Read the model definition and answer for the solid it produces. Units are mm, in the model's axes. A direction names the side the tool comes from. Round coordinates to 2 decimals unless told otherwise and drop trailing zeros. Loops run counter-clockwise (first coordinate to the right, second up) from the corner with the lowest first, then second, coordinate; pieces in that order, holes last. Notation, with made-up numbers: M -40,54.5 L 19,54.5 A20 cw 19,74.5 Z; hole C -31.5,71 d3. An arc over 180 degrees is marked long. Write each question's results on one line, items separated by ' | '.
from build123d import *

# Parameters (mm, degrees)
SALIENTE_EXTRUIR1_DEPTH = 97.7
CROQUIS2_W              = 6.35
CROQUIS2_H              = 85
SALIENTE_EXTRUIR2_DEPTH = 70
CORTAR_EXTRUIR1_DEPTH   = 120
CROQUIS4_R              = 37.5
CROQUIS4_R_2            = 3
CORTAR_EXTRUIR2_DEPTH   = 120
CROQUIS5_W              = 30
CROQUIS5_H              = 18.85
CORTAR_EXTRUIR3_DEPTH   = 120
REDONDEO1_R             = 1
CORTAR_EXTRUIR4_DEPTH   = 110


with BuildPart() as part:
    # Croquis1 → Saliente-Extruir1 (new body)
    with BuildSketch(Plane.XY):
        Polygon((34.307403189, -10.15), (4.307403189, -10.15), (4.307403189, 68.5), (-2.042596811, 68.5), (-2.042596811, -16.5), (34.307403189, -16.5), align=None)
    extrude(amount=SALIENTE_EXTRUIR1_DEPTH)

    # Croquis2 → Saliente-Extruir2 (add)
    with BuildSketch(Plane.ZY.offset(2.042596811)):
        with Locations((3.175, 26)):
            Rectangle(CROQUIS2_W, CROQUIS2_H)
        with Locations((94.525, 26)):
            Rectangle(CROQUIS2_W, CROQUIS2_H)
    extrude(amount=SALIENTE_EXTRUIR2_DEPTH)

    # Croquis3 → Cortar-Extruir1 (cut)
    with BuildSketch(Plane.XY.offset(97.7)):
        Polygon((-72.042596811, -16.5), (-2.042596811, 68.5), (-72.042596811, 68.5), align=None)
    extrude(amount=-CORTAR_EXTRUIR1_DEPTH, mode=Mode.SUBTRACT)

    # Croquis4 → Cortar-Extruir2 (cut)
    with BuildSketch(Plane.ZY.offset(2.042596811)):
        with Locations((48.85, 26)):
            Circle(CROQUIS4_R)
        with Locations((13.85, 62.5)):
            Circle(CROQUIS4_R_2)
        with Locations((13.85, -10.5)):
            Circle(CROQUIS4_R_2)
        with Locations(Location((83.85, -10.5, 0), (0, 0, 6.699765178))):
            Circle(CROQUIS4_R_2)
        with Locations((83.85, 62.5)):
            Circle(CROQUIS4_R_2)
    extrude(amount=-CORTAR_EXTRUIR2_DEPTH, mode=Mode.SUBTRACT)

    # Croquis5 → Cortar-Extruir3 (cut)
    with BuildSketch(Plane(origin=(0, -10.15, 0), x_dir=(1, 0, 0), z_dir=(0, 1, 0))):
        with Locations((19.307403189, -9.425)):
            Rectangle(CROQUIS5_W, CROQUIS5_H)
        with Locations((19.307403189, -88.275)):
            Rectangle(CROQUIS5_W, CROQUIS5_H)
    extrude(amount=-CORTAR_EXTRUIR3_DEPTH, mode=Mode.SUBTRACT)

    # Redondeo1
    redondeo1_edges = [part.edges().sort_by_distance(p)[0] for p in [
        (4.307403189, 68.5, 48.85),
        (4.307403189, -13.325, 18.85),
        (4.307403189, 26, 97.7),
        (4.307403189, -13.325, 78.85),
        (4.307403189, -10.15, 28.864333044),
        (4.307403189, 26, 0),
    ]]
    fillet(redondeo1_edges, radius=REDONDEO1_R)

    # Croquis6 → Cortar-Extruir4 (cut)
    with BuildSketch(Plane(origin=(0, 68.5, 0), x_dir=(1, 0, 0), z_dir=(0, 1, 0))):
        Polygon((4.307403189, -1), (83.921067856, -1), (83.921067856, -107.501215509), (4.307403189, -96.7), align=None)
    extrude(amount=-CORTAR_EXTRUIR4_DEPTH, mode=Mode.SUBTRACT)


solid = part.part
Item 1: For faces 5 (the face through (1.09, -10.61, 40.72)), 6 (the face through (-29, 16, 91.35)), determine the directions among +Z, -Z, +X, -X, +Y, -Y from which every point of the face is accessible in a straight line to the end or side of a thin tool.
Outcome:
face 5: +X, -X | face 6: -X, +Y, -Y
Item 2: Straight lines are drawn through the part: line 1 (Z direction, x = -6, y = 36); line 2 (Y direction, x = 1, z = 83); line 3 (X direction, y = 64, z = 22.5). For each, find the intervals that lie inside material, in ascending order.
Outcome:
line 1: z = 0 to 6.35, 91.35 to 97.7 | line 2: y = -16.5 to -13.38, -7.62 to 10.51, 41.49 to 59.62, 65.38 to 68.5 | line 3: x = -2.04 to 4.31
Item 3: The part is cut by section A-A (z = 48.85). Determine the outline of the cut face in (x, y), plus the area to 3 significant figures.
Outcome:
outline: M -2.04,-16.5 L 4.31,-16.5 L 4.31,-11.5 L -2.04,-11.5 Z; M -2.04,63.5 L 4.31,63.5 L 4.31,67.5 A1 ccw 3.31,68.5 L -2.04,68.5 Z | area: 63.3 mm2
Item 4: The mould has two halves that part along Y. Classify faces 1 (the face through (1.088, -10.368, 10.853)), 2 (the face through (-25, 16, 0)), 3 (the face through (-37.53, 25.41, 94.57)), 4 (the face through (1.088, 62.632, 10.853)): pulls with the +Y half, pulls with the -Y half, needs draft (parallel to the pull), parting line crosses it, or undercut.
Outcome:
face 1: undercut | face 2: needs draft | face 3: pulls with the +Y half | face 4: undercut
Item 5: The part is cut by section D-D (z = 83.85). Determine the outline of the cut face in (x, y).
Outcome:
outline: M -2.04,-16.5 L 4.31,-16.5 L 4.31,-13.5 L -2.04,-13.5 Z; M -2.04,-7.5 L 4.31,-7.5 L 4.31,12.54 L -2.04,12.54 Z; M -2.04,39.46 L 4.31,39.46 L 4.31,59.5 L -2.04,59.5 Z; M -2.04,65.5 L 4.31,65.5 L 4.31,67.5 A1 ccw 3.31,68.5 L -2.04,68.5 Z
Item 6: The part is cut by section C-C (x = -26). Determine the outline of the cut face in (y, z), plus the area to 3 significant figures.
Outcome:
outline: M -16.5,0 L 39.41,0 L 39.41,6.35 L -16.5,6.35 Z; M -16.5,91.35 L 39.41,91.35 L 39.41,97.7 L -16.5,97.7 Z | area: 710 mm2
Item 7: A flat-ended cylindrical pin translates along its axis: pin 1 (10 mm diameter, centred on y = 51.5, z = 73.5, fed in from -X). Find the tip coordinate at first contact, or state that the pin passes through.
Outcome:
pin 1: stops at x = -2.04
Item 8: The part is cut by section B-B (y = -4.5). Determine the outline of the cut face in (x, z).
Outcome:
outline: M -62.16,0 L 3.31,0 A1 ccw 4.31,1 L 4.31,27.03 L -2.04,27.03 L -2.04,6.35 L -62.16,6.35 Z; M -62.16,91.35 L -2.04,91.35 L -2.04,70.67 L 4.31,70.67 L 4.31,96.7 A1 ccw 3.31,97.7 L -62.16,97.7 Z
